from build123d import *

# Parameters (mm, degrees)
CROQUIS4_W            = 3
CROQUIS4_H            = 11
CROQUIS7_W            = 4
CROQUIS7_H            = 8
CORTAR_EXTRUIR1_DEPTH = 7.5
CROQUIS9_W            = 5
CROQUIS9_H            = 8
CORTAR_EXTRUIR2_DEPTH = 7.5
REDONDEO3_R           = 1
CROQUIS10_R           = 2
CORTAR_EXTRUIR3_DEPTH = 7.5


with BuildPart() as part:
    # Croquis4 → Revolución2 (revolve)
    with BuildSketch(Plane(origin=(0, 0, 0), x_dir=(0, 0, -1), z_dir=(1, 0, 0)), mode=Mode.PRIVATE) as revoluci_n2_sk:
        with Locations((-1.5, 5.5)):
            Rectangle(CROQUIS4_W, CROQUIS4_H)
    revolve(revoluci_n2_sk.sketch.rotate(Axis((0, 0, 0), (0, 1, 0)), 180), axis=Axis((0, 0, 0), (0, 1, 0)))

    # Croquis5 → Revolución3 (revolve)
    with BuildSketch(Plane(origin=(0, 0, 0), x_dir=(0, 0, -1), z_dir=(1, 0, 0))):
        with BuildLine():
            Line((0, 20), (0, 11))
            Line((0, 11), (-3, 11))
            ThreePointArc((-3, 11), (-4.74341649, 16.58113883), (0, 20))
        make_face()
    revolve(axis=Axis((0, 20, 0), (0, 1, 0)))

    # Croquis7 → Cortar-Extruir1 (cut, symmetric)
    with BuildSketch(Plane(origin=(0, 0, 0), x_dir=(0, 0, -1), z_dir=(1, 0, 0))):
        with Locations((4, 16)):
            Rectangle(CROQUIS7_W, CROQUIS7_H)
    extrude(amount=CORTAR_EXTRUIR1_DEPTH, both=True, mode=Mode.SUBTRACT)

    # Croquis9 → Cortar-Extruir2 (cut, symmetric)
    with BuildSketch(Plane(origin=(0, 0, 0), x_dir=(0, 0, -1), z_dir=(1, 0, 0))):
        with Locations((-4.5, 16)):
            Rectangle(CROQUIS9_W, CROQUIS9_H)
    extrude(amount=CORTAR_EXTRUIR2_DEPTH, both=True, mode=Mode.SUBTRACT)

    # Redondeo3
    redondeo3_edges = [part.edges().sort_by_distance(p)[0] for p in [
        (0, 12, -2),
        (0, 12, 2),
    ]]
    fillet(redondeo3_edges, radius=REDONDEO3_R)

    # Croquis10 → Cortar-Extruir3 (cut, symmetric)
    with BuildSketch(Plane(origin=(0, 0, 0), x_dir=(-1, 0, 0), z_dir=(0, 0, -1))):
        with Locations((0, 16)):
            Circle(CROQUIS10_R)
    extrude(amount=CORTAR_EXTRUIR3_DEPTH, both=True, mode=Mode.SUBTRACT)


solid = part.part
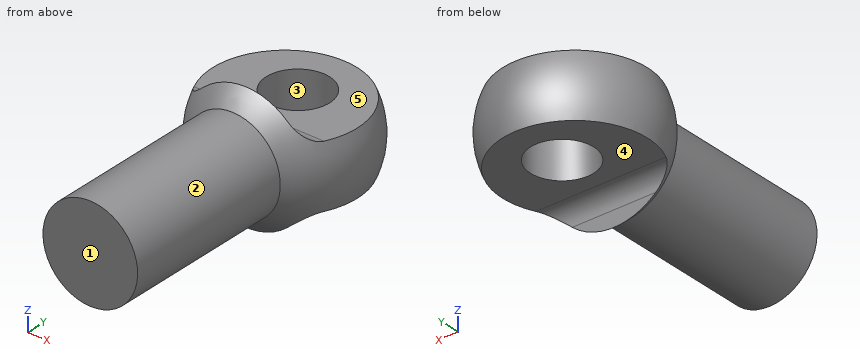
Work out the finished part from the listing and answer in its coordinate system (mm). Face numbers are marked on the shaded views. A direction names the side the tool comes from. Give positions to 0.01 mm unless a question says otherwise; leave off trailing zeros. Order: outer loops, then holes, each group sorted by start corner. A loop starts at its lowest first (then second) coordinate and runs counter-clockwise, first axis right, second up. Notation, with made-up numbers: (23.5, 64) - (67.5, 64) arc R28 ccw to (67.5, 103) - close; hole circle Ø2 at (28, 60). An arc over 180 degrees is marked (long way). Answer as CSV lines item,"result". Start each with the question number.
Q1. The part is cut by section B-B (z = 0). Write down the section's boundary in (x, y), then the cut area to 3 significant figures.
Q2. The mould has two halves that part along Y. Classify the marked faces 1, 2 and 3: +Y half, -Y half, draft (parallel to the pull), parting line (faces both ways), or undercut.
Q3. The part is cut by section A-A (x = 0). Write down the section's boundary in (y, z), then the cut area to 3 significant figures.
Q4. Find the intervals of material crossed by L1, parallel to Y at x = 0, z = -0.2; L2, parallel to Z at x = -0.5, y = 19; L3, parallel to Y at x = -0.25, z = -1, in increasing order. Write a range as [from, to].
Q5. For the marked faces 4 and 5, determine the directions among +Z, -Z, +X, -X, +Y, -Y from which every point of the face is accessible in a straight line to the end or side of a thin tool.
Q6. The part is cut by section C-C (y = 14.5). Write down the section's boundary in (x, z).
Q7. The part is cut by section D-D (x = -1.5). Write down the section's boundary in (y, z).
Q8. Given pin 1 Ø2 at (x, y) = (0.5, 7.5) entering from +Z; pin 2 Ø0.5 at (x, z) = (1, 3.5) entering from +Y; pin 3 Ø3 at (y, z) = (12, -3) entering from -X, each flat-ended and moving along its own axis, determine where each tip first touches the part or whether it passes through.
Check result:
1,outline,"(-3, 0) - (3, 0) - (3, 11) arc R5 ccw (long way) to (-3, 11) - close; hole circle Ø4 at (0, 16)"
1,area,"128 mm²"
2,face 1,"-Y half"
2,face 2,"draft"
2,face 3,"undercut"
3,outline,"(0, -3) - (11, -3) arc R5 ccw to (12, -4) - (12, -3) arc R1 cw to (13, -2) - (14, -2) - (14, 2) - (13, 2) arc R1 cw to (12, 3) - (12, 4) arc R5 ccw to (11, 3) - (0, 3) - close; (18, -2) - (19.58, -2) arc R5 ccw to (19.58, 2) - (18, 2) - close"
3,area,"89.0 mm²"
4,L1,"y = [0, 14], [18, 20]"
4,L2,"z = [-2, 2]"
4,L3,"y = [0, 14.02], [17.98, 19.89]"
5,face 4,"-Z, +X, -X, +Y"
5,face 5,"+Z, +X, -X, +Y"
6,outline,"(-4.56, -2) - (-1.32, -2) - (-1.32, 2) - (-4.56, 2) arc R4.97 ccw to start; (1.32, -2) - (4.56, -2) arc R4.97 ccw to (4.56, 2) - (1.32, 2) - close"
7,outline,"(0, -2.6) - (11, -2.6) arc R4.77 ccw to (12, -3.71) - (12, -3) arc R1 cw to (13, -2) - (14.68, -2) - (14.68, 2) - (13, 2) arc R1 cw to (12, 3) - (12, 3.71) arc R4.77 ccw to (11, 2.6) - (0, 2.6) - close; (17.32, -2) - (19.33, -2) arc R4.77 ccw to (19.33, 2) - (17.32, 2) - close"
8,pin 1,"stops at z = 3"
8,pin 2,"stops at y = 12"
8,pin 3,"stops at x = -4.18"
